For this review, take the finished solid that the model builds, in its own axes (mm). A direction names the side the tool comes from. Give positions to 0.01 mm unless a question says otherwise; leave off trailing zeros. Loops run counter-clockwise (first coordinate to the right, second up) from the corner with the lowest first, then second, coordinate; pieces in that order, holes last.
Autodesk Inventor part; units mm, degrees
ref_plane "YZ Plane" through (0, 0, 0) normal (1, 0, 0) x (0, 1, 0)
ref_plane "XZ Plane" through (0, 0, 0) normal (0, 1, 0) x (-1, 0, 0)
ref_plane "XY Plane" through (0, 0, 0) normal (0, 0, 1) x (1, 0, 0)
sketch "Sketch1" plane through (0, 0, 0) normal (0, 1, 0) x (-1, 0, 0)
  line L0 (4.4017, 8.3575) -> (-0.5983, 8.3575)
  line L1 (-0.5983, 8.3575) -> (-0.5983, -1.6425)
  line L2 (-0.5983, -1.6425) -> (4.4017, -1.6425)
  line L3 (4.4017, -1.6425) -> (4.4017, 8.3575)
  point P0 (0, 0)
  dimension "d0" = 5
  dimension "d1" = 10
extrude "Extrusion1" add sketch "Sketch1" along normal blind 40
sketch "Sketch2" plane through (0.5983, 0, 8.3575) normal (1, 0, 0) x (0, 0, -1)
  line L0 (10, 0) -> (0, 0)
  line L1 (0, 0) -> (10, 0)
  line L2 (10, 0) -> (10, 5)
  line L3 (10, 5) -> (0, 5)
  line L4 (0, 5) -> (0, 0)
  point P0 (8.3575, 0)
  dimension "d4" = 5
extrude "Extrusion2" add sketch "Sketch2" along normal blind 201.85
sketch "Sketch3" plane through (202.4483, 0, 8.3575) normal (1, 0, 0) x (0, 0, -1)
  point P0 (8.3575, 0)
sketch "Sketch4" plane through (0.5983, 5, 8.3575) normal (0, 1, 0) x (1, 0, 0)
  line L0 (-5, 0) -> (201.85, 0)
  line L1 (-5, 10) -> (201.85, 10)
  line L2 (201.85, 0) -> (196.85, 0)
  line L3 (196.85, 0) -> (196.85, 10)
  line L4 (196.85, 10) -> (201.85, 10)
  line L5 (201.85, 10) -> (201.85, 0)
  point P0 (-0.5983, 8.3575)
  point P1 (196.85, 0)
  dimension "d7" = 5
extrude "Extrusion3" add sketch "Sketch4" along normal blind 35
properties part number "tester7.75"
Q1. Consider section A-A on y = 27.5. Give the boundary of the cut face in (x, z), plus the area to 3 significant figures.
Answers:
outline: (-4.4, -1.64) - (0.6, -1.64) - (0.6, 8.36) - (-4.4, 8.36) - close; (197.45, -1.64) - (202.45, -1.64) - (202.45, 8.36) - (197.45, 8.36) - close
area: 100 mm2
Q2. Machinability: for faces 1 (the flat face through (99, 4, 8.358)), 2 (the flat face through (0.598, 22, 3)), which of the approach directions +Z, -Z, +X, -X, +Y, -Y give a long, thin tool a straight path to every point of the face, cutting with its end or side? Answer none if there is none.
Answers:
face 1: +Z, +X, -X, +Y, -Y
face 2: +Z, -Z, +Y
Q3. Consider section B-B on z = 5.5. Give the boundary of the cut face in (x, y).
Answers:
outline: (-4.4, 0) - (202.45, 0) - (202.45, 40) - (197.45, 40) - (197.45, 5) - (0.6, 5) - (0.6, 40) - (-4.4, 40) - close
Q4. Mouldability with a two-part tool opening along X and no side actions: class faces 3 (the flat face through (-4.402, 20, 3)), 4 (the flat face through (197.448, 22, 3)), 5 (the flat face through (202.448, 20, 3)) as +X half, -X half, draft (parallel to the pull), parting line (faces both ways), or undercut.
Answers:
face 3: -X half
face 4: undercut
face 5: +X half
Q5. For pin 1 Ø5 at (x, z) = (69, 2.5) entering from +Y, flat-tipped, find the tip position at first contact; note if it passes through.
Answers:
pin 1: stops at y = 5
Q6. For probe 1 along X at (y, z) = (28.5, 6.5); probe 2 along Y at (x, z) = (61.5, 4), list the stretches that pass through material, from the lowest coordinate up.
Answers:
probe 1: x = -4.4 to 0.6, 197.45 to 202.45
probe 2: y = 0 to 5
Q7. Consider section C-C on x = 118.5. Give the boundary of the cut face in (y, z).
Answers:
outline: (0, -1.64) - (5, -1.64) - (5, 8.36) - (0, 8.36) - close
